Geometry: final body of the model. Coordinates: model frame, mm. A direction names the side the tool comes from. Give positions to 0.01 mm unless a question says otherwise; leave off trailing zeros. Loops run counter-clockwise (first coordinate to the right, second up) from the corner with the lowest first, then second, coordinate; pieces in that order, holes last. Notation, with made-up numbers: (42.25, -25) - (55.25, -25) arc R15 cw to (55.25, -21) - close; hole circle Ø3 at (-40, 39.5). An arc over 180 degrees is marked (long way). Use CSV: the item, a comma, the result in double quotes. Start each with the question number.
```python
from build123d import *

# Parameters (mm, degrees)
SKETCH1_W           = 76.2
SKETCH1_H           = 9.523545078
BOSS_EXTRUDE2_DEPTH = 31.75
SKETCH1_6_R         = 4.5
SKETCH1_6_R_2       = 8.5
BOSS_EXTRUDE3_DEPTH = 6.35


with BuildPart() as part:
    # Sketch1 → Boss-Extrude2 (new, symmetric)
    with BuildSketch(Plane.XY):
        with Locations((0, 44.46410331)):
            Rectangle(SKETCH1_W, SKETCH1_H)
    extrude(amount=BOSS_EXTRUDE2_DEPTH, both=True)

    # Sketch1_6 → Boss-Extrude3 (add, symmetric)
    with BuildSketch(Plane.XY):
        Polygon((-38.1, 39.702330771), (38.1, 39.702330771), (38.1, 12.224), (38.1, -12.224), (-38.1, -12.224), (-38.1, 12.224), align=None)
        with Locations((-19.05, 18.874330771)):
            Circle(SKETCH1_6_R, mode=Mode.SUBTRACT)
        with Locations((19.05, 18.874330771)):
            Circle(SKETCH1_6_R, mode=Mode.SUBTRACT)
        Circle(SKETCH1_6_R_2, mode=Mode.SUBTRACT)
    extrude(amount=BOSS_EXTRUDE3_DEPTH, both=True)


solid = part.part
```
Item 1: Pin query (flat end, axial travel): pin 1 Ø10 at (y, z) = (6.5, 11) entering from -X; pin 2 Ø1.5 at (x, y) = (24.5, 23) entering from -Z; pin 3 Ø15.5 at (x, y) = (18.5, 5.5) entering from +Z; pin 4 Ø12 at (x, z) = (-5.5, 21.5) entering from -Y. Return the tip coordinate at first contact, or that it passes through.
Item 2: Section C-C (z = 3.5). Output: boundary loops of the cut face in (x, y).
Item 3: Reachability of faces 4 (the cylindrical face through (-14.76, 20.23, -0.09)), 5 (the flat face through (1, 14, 6.35)), 6 (the flat face through (-1, 39.702, -19)) from +Z, -Z, +X, -X, +Y, -Y: full face, straight path, thin tool, end or side. Return the list, or none.
Item 4: Section A-A (y = 0). Output: boundary loops of the cut face in (x, z).
Item 5: Section B-B (x = -19.05). Output: boundary loops of the cut face in (y, z), plus the area to 3 significant figures.
Item 6: Mould query, pull axis Y, two halves, no side actions, for faces 1 (the flat face through (-1, 39.702, 19)), 2 (the cylindrical face through (4.57, 7.167, -0.089)), 3 (the flat face through (-38.1, 27, 0)). Classes: pulls with the +Y half, pulls with the -Y half, needs draft (parallel to the pull), parting line crosses it, or undercut.
Item 7: Section D-D (x = 31). Output: boundary loops of the cut face in (y, z).
Item 8: Ray query, probe 1 along Y at (x, z) = (-19.05, -3.5); probe 2 along Y at (x, z) = (17, 6.5); probe 3 along Y at (x, z) = (0, 2.5). Return the intervals inside material, ascending.
Outcome:
1,pin 1,"stops at x = -38.1"
1,pin 2,"stops at z = -6.35"
1,pin 3,"stops at z = 6.35"
1,pin 4,"stops at y = 39.7"
2,outline,"(-38.1, -12.22) - (38.1, -12.22) - (38.1, 49.23) - (-38.1, 49.23) - close; hole circle Ø9 at (-19.05, 18.87); hole circle Ø17 at (0, 0); hole circle Ø9 at (19.05, 18.87)"
3,face 4,"+Z, -Z"
3,face 5,"+Z, +X, -X, -Y"
3,face 6,"-Z, +X, -X, -Y"
4,outline,"(-38.1, -6.35) - (-8.5, -6.35) - (-8.5, 6.35) - (-38.1, 6.35) - close; (8.5, -6.35) - (38.1, -6.35) - (38.1, 6.35) - (8.5, 6.35) - close"
5,outline,"(-12.22, -6.35) - (14.37, -6.35) - (14.37, 6.35) - (-12.22, 6.35) - close; (23.37, -6.35) - (39.7, -6.35) - (39.7, -31.75) - (49.23, -31.75) - (49.23, 31.75) - (39.7, 31.75) - (39.7, 6.35) - (23.37, 6.35) - close"
5,area,"1,150 mm2"
6,face 1,"pulls with the -Y half"
6,face 2,"undercut"
6,face 3,"needs draft"
7,outline,"(-12.22, -6.35) - (39.7, -6.35) - (39.7, -31.75) - (49.23, -31.75) - (49.23, 31.75) - (39.7, 31.75) - (39.7, 6.35) - (-12.22, 6.35) - close"
8,probe 1,"y = -12.22 to 14.37, 23.37 to 49.23"
8,probe 2,"y = 39.7 to 49.23"
8,probe 3,"y = -12.22 to -8.5, 8.5 to 49.23"
